Geometry: final body of the model. Coordinates: model frame, mm. Face numbers are marked on the shaded views. A direction names the side the tool comes from. Give positions to 0.01 mm unless a question says otherwise; leave off trailing zeros. Write each loop counter-clockwise with the first axis right and the second up, starting at its lowest first coordinate (ties: lowest second). Pieces come first, ordered by that corner, then holes. Notation, with made-up numbers: (-13.75, 14) -> (36.25, 14) arc R14 cw to (36.25, 22) -> close; hole circle Ø7 at (23, 33.5). An arc over 180 degrees is marked (long way). Answer in a Markdown table with one row per item. Add a question column.
from build123d import *

# Parameters (mm, degrees)
F1_DEPTH = 25


with BuildPart() as f1:
    # F0 (on Front) → F1 (new body)
    with BuildSketch(Plane.XZ):
        with BuildLine():
            ThreePointArc((1.99609, 15.875), (0, 16), (-1.99609, 15.875))
            ThreePointArc((-1.99609, 15.875), (-2.778371, 15.756924), (-3.553859, 15.600323))
            ThreePointArc((-3.553859, 15.600323), (-5.472322, 15.035082), (-7.305281, 14.234917))
            ThreePointArc((-7.305281, 14.234917), (-8, 13.856406), (-8.67516, 13.444017))
            ThreePointArc((-8.67516, 13.444017), (-10.284602, 12.256711), (-11.733347, 10.877894))
            ThreePointArc((-11.733347, 10.877894), (-12.256711, 10.284602), (-12.750108, 9.666165))
            ThreePointArc((-12.750108, 9.666165), (-13.856406, 8), (-14.746198, 6.208835))
            ThreePointArc((-14.746198, 6.208835), (-15.035082, 5.472322), (-15.287206, 4.72243))
            ThreePointArc((-15.287206, 4.72243), (-15.756924, 2.778371), (-15.98044, 0.7909))
            ThreePointArc((-15.98044, 0.7909), (-16, 0), (-15.98044, -0.7909))
            ThreePointArc((-15.98044, -0.7909), (-15.756924, -2.778371), (-15.287206, -4.72243))
            ThreePointArc((-15.287206, -4.72243), (-15.035082, -5.472322), (-14.746198, -6.208835))
            ThreePointArc((-14.746198, -6.208835), (-13.856406, -8), (-12.750108, -9.666165))
            ThreePointArc((-12.750108, -9.666165), (-12.256711, -10.284602), (-11.733347, -10.877894))
            ThreePointArc((-11.733347, -10.877894), (-10.284602, -12.256711), (-8.67516, -13.444017))
            ThreePointArc((-8.67516, -13.444017), (-8, -13.856406), (-7.305281, -14.234917))
            ThreePointArc((-7.305281, -14.234917), (-5.472322, -15.035082), (-3.553859, -15.600323))
            ThreePointArc((-3.553859, -15.600323), (-2.778371, -15.756924), (-1.99609, -15.875))
            ThreePointArc((-1.99609, -15.875), (-1, -15.968719), (0, -16))
            ThreePointArc((0, -16), (1, -15.968719), (1.99609, -15.875))
            ThreePointArc((1.99609, -15.875), (2.778371, -15.756924), (3.553859, -15.600323))
            ThreePointArc((3.553859, -15.600323), (5.472322, -15.035082), (7.305281, -14.234917))
            ThreePointArc((7.305281, -14.234917), (8, -13.856406), (8.67516, -13.444017))
            ThreePointArc((8.67516, -13.444017), (10.284602, -12.256711), (11.733347, -10.877894))
            ThreePointArc((11.733347, -10.877894), (12.256711, -10.284602), (12.750108, -9.666165))
            ThreePointArc((12.750108, -9.666165), (13.856406, -8), (14.746198, -6.208835))
            ThreePointArc((14.746198, -6.208835), (15.035082, -5.472322), (15.287206, -4.72243))
            ThreePointArc((15.287206, -4.72243), (15.756924, -2.778371), (15.98044, -0.7909))
            ThreePointArc((15.98044, -0.7909), (16, 0), (15.98044, 0.7909))
            ThreePointArc((15.98044, 0.7909), (15.756924, 2.778371), (15.287206, 4.72243))
            ThreePointArc((15.287206, 4.72243), (15.035082, 5.472322), (14.746198, 6.208835))
            ThreePointArc((14.746198, 6.208835), (13.856406, 8), (12.750108, 9.666165))
            ThreePointArc((12.750108, 9.666165), (12.256711, 10.284602), (11.733347, 10.877894))
            ThreePointArc((11.733347, 10.877894), (10.284602, 12.256711), (8.67516, 13.444017))
            ThreePointArc((8.67516, 13.444017), (8, 13.856406), (7.305281, 14.234917))
            ThreePointArc((7.305281, 14.234917), (5.472322, 15.035082), (3.553859, 15.600323))
            ThreePointArc((3.553859, 15.600323), (2.778371, 15.756924), (1.99609, 15.875))
        make_face()
        Polygon((-2.12708, 5.013831), (3.278565, 4.349021), (5.405645, -0.66481), (2.12708, -5.013831), (-3.278565, -4.349021), (-5.405645, 0.66481), align=None, mode=Mode.SUBTRACT)
        with BuildLine():
            Line((6.156363, 16.914467), (3.553859, 15.600323))
            ThreePointArc((3.553859, 15.600323), (5.472322, 15.035082), (7.305281, 14.234917))
            Line((7.305281, 14.234917), (6.156363, 16.914467))
        make_face()
        with BuildLine():
            Line((0, 18), (-1.99609, 15.875))
            ThreePointArc((-1.99609, 15.875), (0, 16), (1.99609, 15.875))
            Line((1.99609, 15.875), (0, 18))
        make_face()
        with BuildLine():
            ThreePointArc((-7.305281, 14.234917), (-5.472322, 15.035082), (-3.553859, 15.600323))
            Line((-3.553859, 15.600323), (-6.156363, 16.914467))
            Line((-6.156363, 16.914467), (-7.305281, 14.234917))
        make_face()
        with BuildLine():
            ThreePointArc((-11.733347, 10.877894), (-10.284602, 12.256711), (-8.67516, 13.444017))
            Line((-8.67516, 13.444017), (-11.570177, 13.7888))
            Line((-11.570177, 13.7888), (-11.733347, 10.877894))
        make_face()
        with BuildLine():
            ThreePointArc((-14.746198, 6.208835), (-13.856406, 8), (-12.750108, 9.666165))
            Line((-12.750108, 9.666165), (-15.588457, 9))
            Line((-15.588457, 9), (-14.746198, 6.208835))
        make_face()
        with BuildLine():
            ThreePointArc((-15.98044, 0.7909), (-15.756924, 2.778371), (-15.287206, 4.72243))
            Line((-15.287206, 4.72243), (-17.72654, 3.125667))
            Line((-17.72654, 3.125667), (-15.98044, 0.7909))
        make_face()
        with BuildLine():
            ThreePointArc((-15.287206, -4.72243), (-15.756924, -2.778371), (-15.98044, -0.7909))
            Line((-15.98044, -0.7909), (-17.72654, -3.125667))
            Line((-17.72654, -3.125667), (-15.287206, -4.72243))
        make_face()
        with BuildLine():
            ThreePointArc((-12.750108, -9.666165), (-13.856406, -8), (-14.746198, -6.208835))
            Line((-14.746198, -6.208835), (-15.588457, -9))
            Line((-15.588457, -9), (-12.750108, -9.666165))
        make_face()
        with BuildLine():
            ThreePointArc((-8.67516, -13.444017), (-10.284602, -12.256711), (-11.733347, -10.877894))
            Line((-11.733347, -10.877894), (-11.570177, -13.7888))
            Line((-11.570177, -13.7888), (-8.67516, -13.444017))
        make_face()
        with BuildLine():
            ThreePointArc((-3.553859, -15.600323), (-5.472322, -15.035082), (-7.305281, -14.234917))
            Line((-7.305281, -14.234917), (-6.156363, -16.914467))
            Line((-6.156363, -16.914467), (-3.553859, -15.600323))
        make_face()
        with BuildLine():
            ThreePointArc((0, -16), (-1, -15.968719), (-1.99609, -15.875))
            Line((-1.99609, -15.875), (0, -18))
            Line((0, -18), (1.99609, -15.875))
            ThreePointArc((1.99609, -15.875), (1, -15.968719), (0, -16))
        make_face()
        with BuildLine():
            Line((6.156363, -16.914467), (7.305281, -14.234917))
            ThreePointArc((7.305281, -14.234917), (5.472322, -15.035082), (3.553859, -15.600323))
            Line((3.553859, -15.600323), (6.156363, -16.914467))
        make_face()
        with BuildLine():
            Line((15.588457, -9), (14.746198, -6.208835))
            ThreePointArc((14.746198, -6.208835), (13.856406, -8), (12.750108, -9.666165))
            Line((12.750108, -9.666165), (15.588457, -9))
        make_face()
        with BuildLine():
            Line((17.72654, -3.125667), (15.98044, -0.7909))
            ThreePointArc((15.98044, -0.7909), (15.756924, -2.778371), (15.287206, -4.72243))
            Line((15.287206, -4.72243), (17.72654, -3.125667))
        make_face()
        with BuildLine():
            Line((17.72654, 3.125667), (15.287206, 4.72243))
            ThreePointArc((15.287206, 4.72243), (15.756924, 2.778371), (15.98044, 0.7909))
            Line((15.98044, 0.7909), (17.72654, 3.125667))
        make_face()
        with BuildLine():
            Line((15.588457, 9), (12.750108, 9.666165))
            ThreePointArc((12.750108, 9.666165), (13.856406, 8), (14.746198, 6.208835))
            Line((14.746198, 6.208835), (15.588457, 9))
        make_face()
        with BuildLine():
            Line((11.570177, 13.7888), (8.67516, 13.444017))
            ThreePointArc((8.67516, 13.444017), (10.284602, 12.256711), (11.733347, 10.877894))
            Line((11.733347, 10.877894), (11.570177, 13.7888))
        make_face()
        with BuildLine():
            Line((11.570177, -13.7888), (11.733347, -10.877894))
            ThreePointArc((11.733347, -10.877894), (10.284602, -12.256711), (8.67516, -13.444017))
            Line((8.67516, -13.444017), (11.570177, -13.7888))
        make_face()
    extrude(amount=F1_DEPTH)


solid = f1.part
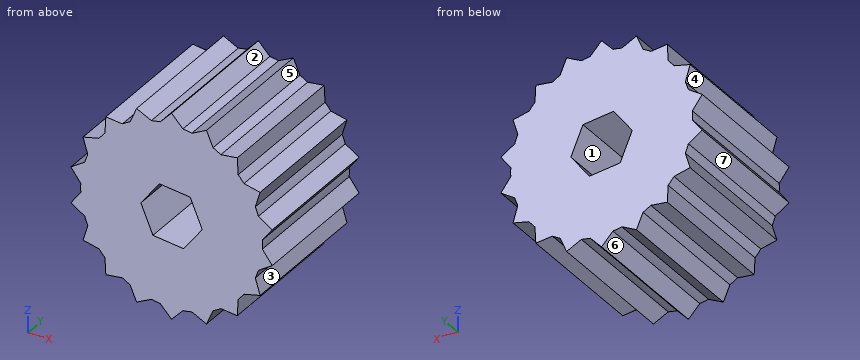
Q1. Section A-A on x = -4.5. Return loops of the section in (y, z).
Q2. Access query for the marked faces 1, 2, 3 and 4. Directions: +Z, -Z, +X, -X, +Y, -Y. A direction counts if a zero-diameter tool reaches every point of the face in a straight line with its end or side. Return the directions, or none.
Q3. Contact query for flat-ended pins moving along their axis: pin 1 Ø12 at (y, z) = (-22.5, 9.5) entering from +X; pin 2 Ø1.5 at (x, y) = (-1, -22) entering from +Z; pin 3 Ø12 at (y, z) = (-14.5, 9.5) entering from -X. Output: stop coordinate, or through.
Q4. Section C-C on x = -9.5. Return loops of the section in (y, z).
Q5. Line query: probe 1 along X at (y, z) = (-18, -16); probe 2 along X at (y, z) = (-6.25, 0); probe 3 along Z at (x, y) = (-0.5, -4.5). Output: solid intervals per line, ascending. Write a range as from..to.
Q6. Pull-direction query (X, two-part tool) for the marked faces 5, 6 and 7; classes: +X half, -X half, draft (parallel to the pull), parting line (faces both ways), or undercut.
Q7. Section D-D on z = -7. Return loops of the section in (x, y).
Q8. Section B-B on z = 2.5. Return loops of the section in (x, y), and give its area (3 significant figures).
Checks:
| question | item | result |
|---|---|---|
| 1 | outline | (-25, -16.08) -> (0, -16.08) -> (0, -1.47) -> (-25, -1.47) -> close; (-25, 1.87) -> (0, 1.87) -> (0, 16.08) -> (-25, 16.08) -> close |
| 2 | face 1 | +Y, -Y |
| 2 | face 2 | +Z, +Y, -Y |
| 2 | face 3 | +X, +Y, -Y |
| 2 | face 4 | -X, +Y, -Y |
| 3 | pin 1 | x = 17.15 |
| 3 | pin 2 | z = 17.73 |
| 3 | pin 3 | x = -17.15 |
| 4 | outline | (-25, -13.54) -> (0, -13.54) -> (0, 13.54) -> (-25, 13.54) -> close |
| 5 | probe 1 | -6.55..-4.35, -1.88..1.88, 4.35..6.55 |
| 5 | probe 2 | -16..-5.12, 5.12..16 |
| 5 | probe 3 | -17.47..-4.69, 4.81..17.47 |
| 6 | face 5 | +X half |
| 6 | face 6 | undercut |
| 6 | face 7 | -X half |
| 7 | outline | (-14.98, -25) -> (14.98, -25) -> (14.98, 0) -> (-14.98, 0) -> close |
| 8 | outline | (-17.26, -25) -> (-4.02, -25) -> (-4.02, 0) -> (-17.26, 0) -> close; (4.06, -25) -> (17.26, -25) -> (17.26, 0) -> (4.06, 0) -> close |
| 8 | area | 661 mm^2 |
